Design review of the part built by this model. Coordinates are the model's own, in mm. Coordinates: 2 decimals unless noted, no trailing zeros. Order: outer loops, then holes, each group sorted by start corner. A loop starts at its lowest first (then second) coordinate and runs counter-clockwise, first axis right, second up. Notation, with made-up numbers: M 30.25,-9.5 L 61.25,-9.5 A23 ccw 61.25,21.5 Z; hole C -1.5,81 d2. An arc over 180 degrees is marked long. Answer as a JSON object with one key per item and string values.
Autodesk Inventor part; units mm, degrees
ref_plane "YZ Plane" through (0, 0, 0) normal (1, 0, 0) x (0, 1, 0)
ref_plane "XZ Plane" through (0, 0, 0) normal (0, 1, 0) x (-1, 0, 0)
ref_plane "XY Plane" through (0, 0, 0) normal (0, 0, 1) x (1, 0, 0)
sketch "Sketch1" plane through (0, 0, 0) normal (0, 1, 0) x (-1, 0, 0)
  circle A0 centre (0, 0) radius 10
  dimension "d0" = 20
extrude "Extrusion1" add sketch "Sketch1" along normal blind 22.5
sketch "Sketch2" plane through (0, 0, 0) normal (0, -1, 0) x (1, 0, 0)
  circle A0 centre (0, 0) radius 6
  dimension "d3" = 12
extrude "Extrusion2" cut sketch "Sketch2" against normal through all
sketch "Sketch3" plane through (0, 0, 0) normal (0, -1, 0) x (1, 0, 0)
  circle A0 centre (0, 0) radius 10
  circle A1 centre (0, 0) radius 12.5
  dimension "d6" = 25
extrude "Extrusion3" add sketch "Sketch3" against normal blind 5
fillet "Fillet1" radius 2 1 edges at (10, 22.5, 0)
properties part number "Bushing_stempel" material "Brass, Soft Yellow"
1) To check wall thickness, follow L1, parallel to Z at x = 0, y = 16.75; L2, parallel to Z at x = -1.75, y = 2.5; L3, parallel to Y at x = 1.25, z = -8. State the ranges of each line that lie inside material, in increasing order.
Taken from the geometry:
{"L1": "z = -10 to -6, 6 to 10", "L2": "z = -12.38 to -5.74, 5.74 to 12.38", "L3": "y = 0 to 22.5"}
2) Add section C-C (y = 6.5). State the section outline as (x, z) points.
Taken from the geometry:
{"outline": "C 0,0 d20; hole C 0,0 d12"}
3) Mouldability with a two-part tool opening along X and no side actions: class faces 1 (the cylindrical face through (2.17, 12.64, 9.76)), 2 (the cylindrical face through (-6, 11, 0)), 3 (the flat face through (-0.1, 5, 10.2)) as released by +X, released by -X, zero draft, split by the parting line, or undercut.
Taken from the geometry:
{"face 1": "split by the parting line", "face 2": "undercut", "face 3": "zero draft"}
4) Add section D-D (x = -10.75). State the section outline as (y, z) points, and give its area (3 significant figures).
Taken from the geometry:
{"outline": "M 0,-6.38 L 5,-6.38 L 5,6.38 L 0,6.38 Z", "area": "63.8 mm2"}
5) Insertion check: pin 1 Ø2 at (y, z) = (16.5, -8.5) entering from +X; pin 2 Ø10 at (y, z) = (19.5, 0.5) entering from +X; pin 3 Ø3 at (x, y) = (-7.5, 5) entering from +Z; pin 4 Ø9.5 at (x, z) = (0, 0) entering from -Y. Each pin has a flat end and moves straight along its axis. Give the tip position at first contact, or say it passes through.
Taken from the geometry:
{"pin 1": "stops at x = 6.61", "pin 2": "stops at x = 10", "pin 3": "stops at z = 10.97", "pin 4": "passes through"}
6) Add section A-A (z = 0). State the section outline as (x, y) points, and give its area (3 significant figures).
Taken from the geometry:
{"outline": "M -12.5,0 L -6,0 L -6,22.5 L -8,22.5 A2 ccw -10,20.5 L -10,5 L -12.5,5 Z; M 6,0 L 12.5,0 L 12.5,5 L 10,5 L 10,20.5 A2 ccw 8,22.5 L 6,22.5 Z", "area": "203 mm2"}
7) Add section B-B (x = 0). State the section outline as (y, z) points, and give its area (3 significant figures).
Taken from the geometry:
{"outline": "M 0,-12.5 L 5,-12.5 L 5,-10 L 20.5,-10 A2 ccw 22.5,-8 L 22.5,-6 L 0,-6 Z; M 0,6 L 22.5,6 L 22.5,8 A2 ccw 20.5,10 L 5,10 L 5,12.5 L 0,12.5 Z", "area": "203 mm2"}
